Input: part model. Units: mm. Frame: model coordinates. A direction names the side the tool comes from. Coordinates: 2 decimals unless noted, no trailing zeros. Order: outer loops, then holes, each group sorted by start corner. A loop starts at its lowest first (then second) coordinate and runs counter-clockwise, first axis right, second up. Notation, with made-up numbers: (84, 59) -> (140, 59) arc R30 cw to (140, 81) -> close; hole circle Ø9 at (56.25, 43). An arc over 180 degrees is marked (long way). Use CSV: the item, a comma, the result in double quotes. Start each with the question number.
```python
from build123d import *

# Parameters (mm, degrees)
SKETCH1_W               = 86.36
SKETCH1_H               = 38.1
SKETCH1_W_2             = 76.2
SKETCH1_H_2             = 27.94
BOSS_EXTRUDE1_DEPTH     = 127
SKETCH2_R               = 9.000000018
SKETCH2_R_2             = 3.175
CUT_EXTRUDE1_DEPTH      = 156.521858271
SKETCH3_R               = 3.81
CUT_EXTRUDE2_DEPTH      = 158.090324336
CUT_EXTRUDE2_DEPTH_BACK = 158.090324336
SKETCH4_R               = 6.35
SKETCH4_R_2             = 3.175
BOSS_EXTRUDE2_DEPTH     = 4.385
SKETCH5_R               = 6.35
SKETCH5_R_2             = 3.175
BOSS_EXTRUDE3_DEPTH     = 4.38500012
SKETCH6_R               = 12.7
SKETCH6_R_2             = 6.5
BOSS_EXTRUDE4_DEPTH     = 2.54
SKETCH7_R               = 12.7
SKETCH7_R_2             = 6.5
BOSS_EXTRUDE5_DEPTH     = 2.54


with BuildPart() as part:
    # Sketch1 → Boss-Extrude1 (new body)
    with BuildSketch(Plane(origin=(0, 0, 0), x_dir=(1, 0, 0), z_dir=(0, 1, 0))):
        with Locations((38.1, 13.97)):
            Rectangle(SKETCH1_W, SKETCH1_H)
        with Locations((38.1, 13.97)):
            Rectangle(SKETCH1_W_2, SKETCH1_H_2, mode=Mode.SUBTRACT)
    extrude(amount=BOSS_EXTRUDE1_DEPTH)

    # Sketch2 → Cut-Extrude1 (cut, through all)
    with BuildSketch(Plane.XY.offset(5.08)):
        with Locations((38.1, 88.9)):
            Circle(SKETCH2_R)
        with Locations((17.833355107, 41.428109825)):
            Circle(SKETCH2_R_2)
    extrude(amount=-CUT_EXTRUDE1_DEPTH, mode=Mode.SUBTRACT)

    # Sketch3 → Cut-Extrude2 (cut, two sides)
    with BuildSketch(Plane(origin=(81.28, 0, 0), x_dir=(0, 0, -1), z_dir=(1, 0, 0))) as cut_extrude2_sk:
        with Locations(Location((13.97, 114.3, 0), (0, 0, 180))):
            Circle(SKETCH3_R)
        with Locations(Location((13.97, 25.4, 0), (0, 0, 180))):
            Circle(SKETCH3_R)
    extrude(amount=CUT_EXTRUDE2_DEPTH, mode=Mode.SUBTRACT)
    extrude(cut_extrude2_sk.sketch, amount=-CUT_EXTRUDE2_DEPTH_BACK, mode=Mode.SUBTRACT)

    # Sketch4 → Boss-Extrude2 (add)
    with BuildSketch(Plane(origin=(0, 0, -33.02), x_dir=(-1, 0, 0), z_dir=(0, 0, -1))):
        with Locations(Location((-17.833355107, 41.428109825, 0), (0, 0, 180))):
            Circle(SKETCH4_R)
        with Locations(Location((-17.833355107, 41.428109825, 0), (0, 0, 180))):
            Circle(SKETCH4_R_2, mode=Mode.SUBTRACT)
    extrude(amount=BOSS_EXTRUDE2_DEPTH)

    # Sketch5 → Boss-Extrude3 (add)
    with BuildSketch(Plane.XY.offset(5.08)):
        with Locations((17.833355107, 41.428109825)):
            Circle(SKETCH5_R)
        with Locations((17.833355107, 41.428109825)):
            Circle(SKETCH5_R_2, mode=Mode.SUBTRACT)
    extrude(amount=BOSS_EXTRUDE3_DEPTH)

    # Sketch6 → Boss-Extrude4 (add)
    with BuildSketch(Plane.XY.offset(5.08)):
        with Locations(Location((38.1, 88.9, 0), (0, 0, 180))):
            Circle(SKETCH6_R)
        with Locations((38.1, 88.9)):
            Circle(SKETCH6_R_2, mode=Mode.SUBTRACT)
    extrude(amount=BOSS_EXTRUDE4_DEPTH)

    # Sketch7 → Boss-Extrude5 (add)
    with BuildSketch(Plane(origin=(0, 0, -33.02), x_dir=(-1, 0, 0), z_dir=(0, 0, -1))):
        with Locations((-38.1, 88.9)):
            Circle(SKETCH7_R)
        with Locations(Location((-38.1, 88.9, 0), (0, 0, 180))):
            Circle(SKETCH7_R_2, mode=Mode.SUBTRACT)
    extrude(amount=BOSS_EXTRUDE5_DEPTH)


solid = part.part
```
1. Contact query for flat-ended pins moving along their axis: P1, Ø12.5, axis at x = 41.5, y = 88, coming from the -Z side; P2, Ø2, axis at x = 55.5, y = 67, coming from the -Z side; P3, Ø4, axis at x = 23, y = 57.5, coming from the +Z side; P4, Ø8.5, axis at x = 17.83, y = 41.43, coming from the -Z side (3 decimals). Output: stop coordinate, or through.
2. Section B-B on x = 38.1. State how many separate pieces and enclosed holes the cut face has, then the cut area to 3 significant figures.
3. Access query for faces 1 (the face through (76.2, 63, -14)), 2 (the face through (42.94, 96.49, -30.44)), 3 (the face through (37.254, 95.345, 6.332)), 4 (the face through (39.753, 76.308, 6.332)). Directions: +Z, -Z, +X, -X, +Y, -Y. A direction counts if a zero-diameter tool reaches every point of the face in a straight line with its end or side. Return the directions, or none.
4. Material intervals for line 1 along X through (y, z) = (108.5, -14.5); line 2 along Z through (x, y) = (31, 118.5); line 3 along Y through (x, z) = (38.1, -34.45), sorted ascending.
5. Pull-direction query (Y, two-part tool) for faces 5 (the face through (15.493, 39.282, -32.606)), 6 (the face through (31.5, 127, -28.2)), 7 (the face through (39.753, 101.492, -34.272)); classes: released by +Y, released by -Y, zero draft, split by the parting line, or undercut.
6. Section A-A on z = -13.97. Return loops of the section in (x, y), then the cut area to 3 significant figures.
7. Section D-D on y = 105. Return loops of the section in (x, z).
Values follow:
1,P1,"stops at z = -35.56"
1,P2,"stops at z = -33.02"
1,P3,"stops at z = 5.08"
1,P4,"stops at z = -37.405"
2,separate pieces,"4"
2,enclosed holes,"0"
2,area,"1,170 mm2"
3,face 1,"+Y, -Y"
3,face 2,"none"
3,face 3,"+Z, -Z"
3,face 4,"+Z"
4,line 1,"x = -5.08 to 0, 76.2 to 81.28"
4,line 2,"z = -33.02 to -27.94, 0 to 5.08"
4,line 3,"y = 76.2 to 82.4, 95.4 to 101.6"
5,face 5,"undercut"
5,face 6,"released by +Y"
5,face 7,"split by the parting line"
6,outline,"(-5.08, 0) -> (0, 0) -> (0, 21.59) -> (-5.08, 21.59) -> close; (-5.08, 29.21) -> (0, 29.21) -> (0, 110.49) -> (-5.08, 110.49) -> close; (-5.08, 118.11) -> (0, 118.11) -> (0, 127) -> (-5.08, 127) -> close; (76.2, 0) -> (81.28, 0) -> (81.28, 21.59) -> (76.2, 21.59) -> close; (76.2, 29.21) -> (81.28, 29.21) -> (81.28, 110.49) -> (76.2, 110.49) -> close; (76.2, 118.11) -> (81.28, 118.11) -> (81.28, 127) -> (76.2, 127) -> close"
6,area,"1,140 mm2"
7,outline,"(-5.08, -33.02) -> (81.28, -33.02) -> (81.28, 5.08) -> (-5.08, 5.08) -> close; hole (0, -27.94) -> (76.2, -27.94) -> (76.2, 0) -> (0, 0) -> close"
